Autodesk Inventor part; units mm, degrees
ref_plane "YZ Plane" through (0, 0, 0) normal (1, 0, 0) x (0, 1, 0)
ref_plane "XZ Plane" through (0, 0, 0) normal (0, 1, 0) x (-1, 0, 0)
ref_plane "XY Plane" through (0, 0, 0) normal (0, 0, 1) x (1, 0, 0)
sketch "Pole Base Profile" plane through (0, 0, 0) normal (0, 1, 0) x (-1, 0, 0)
  line L0 (3.725, 2.7) -> (-3.725, 2.7)
  line L1 (-3.725, 2.7) -> (-3.725, -2.7)
  line L2 (-3.725, -2.7) -> (3.725, -2.7)
  line L3 (3.725, -2.7) -> (3.725, 2.7)
  line L4 (3.725, 2.7) -> (-3.725, -2.7) construction
  line L5 (-3.725, 2.7) -> (3.725, -2.7) construction
  point P0 (0, 0)
  dimension "d0" = 7.45
  dimension "d1" = 5.4
extrude "Pole Base" add sketch "Pole Base Profile" along normal blind 3
sketch "Cross Base" plane through (0, 3, 0) normal (0, 1, 0) x (1, 0, 0)
  line L0 (-0.55, -2.075) -> (0.55, -2.075)
  line L1 (0.55, -2.075) -> (0.55, 2.075)
  line L2 (0.55, 2.075) -> (-0.55, 2.075)
  line L3 (-0.55, 2.075) -> (-0.55, -2.075)
  line L4 (-0.55, -2.075) -> (0.55, 2.075) construction
  line L5 (0.55, -2.075) -> (-0.55, 2.075) construction
  line L6 (-2.075, -0.55) -> (2.075, -0.55)
  line L7 (2.075, -0.55) -> (2.075, 0.55)
  line L8 (2.075, 0.55) -> (-2.075, 0.55)
  line L9 (-2.075, 0.55) -> (-2.075, -0.55)
  line L10 (-2.075, -0.55) -> (2.075, 0.55) construction
  line L11 (2.075, -0.55) -> (-2.075, 0.55) construction
  point P0 (0, 0)
  dimension "d12" = 1.1
  dimension "d13" = 4.15
  dimension "d14" = 4.15
  dimension "d15" = 1.1
extrude "Pole" add sketch "Cross Base" along normal blind 3.6
fillet "Pole Rounding" radius 0.25 8 edges at (2.075, 4.8, 0.55) (0.55, 4.8, 2.075) (-0.55, 4.8, 2.075) (-2.075, 4.8, 0.55) (-2.075, 4.8, -0.55) (-0.55, 4.8, -2.075) (0.55, 4.8, -2.075) (2.075, 4.8, -0.55)
fillet "Base Rounding" radius 0.3 4 edges at (-3.725, 3, 0) (0, 3, -2.7) (0, 3, 2.7) (3.725, 3, 0)
sketch "Top Center Point" plane through (0, 6.6, 0) normal (0, 1, 0) x (1, 0, 0)
  point P0 (0, 0)
equation "\"d0\" = s_polebl"
equation "\"d1\" = s_polebw"
equation "\"d12\" = k_cmxw"
equation "\"d13\" = k_cmxl"
equation "\"d14\" = d13"
equation "\"d15\" = d12"
equation "\"d8\" = s_poleh"
equation "\"k_width\" = 18"
equation "\"k_height\" = 16.5"
equation "\"k_taper1\" = 1.5"
equation "\"k_taper2\" = 0.5"
equation "\"k_radius\" = 6"
equation "\"k_wthick\" = 1.5"
equation "\"k_ribthick\" = 1.5"
equation "\"k_ribheight\" = 5"
equation "\"k_poleoff\" = 2.25"
equation "\"k_poledia\" = 5.3"
equation "\"k_cmxw\" = 1.1"
equation "\"k_cmxl\" = 4.15"
equation "\"s_bwidth\" = 14.4"
equation "\"s_poleh\" = 3.6"
equation "\"s_polebw\" = 5.4"
equation "\"s_polebl\" = 7.45"
equation "\"b_rshift\" = 49.5"
equation "\"b_height\" = 77"
equation "\"b_tab\" = 27"
equation "\"b_lshift\" = 40.5"
equation "\"b_space\" = 117"
equation "\"b_caps\" = 31.5"
equation "\"b_pad\" = 1"
equation "\"b_width\" = 285"
equation "\"b_ctrl\" = 22.5"
equation "\"k_staper\" = 1"
equation "\"k_ltaper\" = 1.5"
equation "\"k_sradius\" = 4"
equation "\"k_lradius\" = 6"
equation "\"k_height_t\" = 16"
equation "\"k_height_low\" = 15"
equation "\"k_taper_wide\" = 1.5"
equation "\"k_taper_thin\" = 0.0001"
equation "\"k_shortening\" = 4.5"
equation "\"k_cmxd\" = 4"
equation "\"k_taper_side\" = 0.5"
properties part number "keyswitch-pole_cherrymx"
Here's how the part is built. I have some questions about the finished solid (model axes, mm). A direction names the side the tool comes from. Round coordinates to 2 decimals unless told otherwise and drop trailing zeros. Loops run counter-clockwise (first coordinate to the right, second up) from the corner with the lowest first, then second, coordinate; pieces in that order, holes last.
1. If we section it at D-D on x = -3: Write out the boundary of the cut face in (y, z), plus the area to 3 significant figures.
Answer list:
outline: (0, -2.7) - (2.7, -2.7) arc R0.3 ccw to (3, -2.4) - (3, 2.4) arc R0.3 ccw to (2.7, 2.7) - (0, 2.7) - close
area: 16.2 mm2
2. If we section it at C-C on z = -0.05: Write out the boundary of the cut face in (x, y) (3 decimals).
Answer list:
outline: (-3.725, 0) - (3.725, 0) - (3.725, 2.7) arc R0.3 ccw to (3.425, 3) - (2.075, 3) - (2.075, 6.6) - (-2.075, 6.6) - (-2.075, 3) - (-3.425, 3) arc R0.3 ccw to (-3.725, 2.7) - close
3. Which directions (+Z, -Z, +X, -X, +Y, -Y) give clear straight access to the entire face, cutting with the end or side of a thin tool? Please do faces 1 (the face through (1, 5, -0.55)), 2 (the face through (-1, 5, 0.55)), 3 (the face through (0.55, 5, 1)), 4 (the face through (-1, 5, -0.55)), 5 (the face through (1, 3, 1)).
Answer list:
face 1: -Z, +X, +Y
face 2: +Z, -X, +Y
face 3: +Z, +X, +Y
face 4: -Z, -X, +Y
face 5: +Y
4. If we section it at B-B on y = 5: Write out the boundary of the cut face in (x, z) (3 decimals).
Answer list:
outline: (-2.075, -0.3) arc R0.25 ccw to (-1.825, -0.55) - (-0.55, -0.55) - (-0.55, -1.825) arc R0.25 ccw to (-0.3, -2.075) - (0.3, -2.075) arc R0.25 ccw to (0.55, -1.825) - (0.55, -0.55) - (1.825, -0.55) arc R0.25 ccw to (2.075, -0.3) - (2.075, 0.3) arc R0.25 ccw to (1.825, 0.55) - (0.55, 0.55) - (0.55, 1.825) arc R0.25 ccw to (0.3, 2.075) - (-0.3, 2.075) arc R0.25 ccw to (-0.55, 1.825) - (-0.55, 0.55) - (-1.825, 0.55) arc R0.25 ccw to (-2.075, 0.3) - close
5. For P1, Ø0.5, axis at y = 5, z = 0, coming from the +X side (3 decimals); P2, Ø1, axis at x = 1.5, y = 4.5, coming from the -Z side; P3, Ø3, axis at x = 0, y = 3, coming from the -Z side; P4, Ø1.5, axis at x = 0.5, y = 5.5, coming from the -Z side (3 decimals), each with a flat end and sliding along its axis, tell me the tip position at first contact or that it passes through.
Answer list:
P1: stops at x = 2.075
P2: stops at z = -0.55
P3: stops at z = -2.7
P4: stops at z = -2.075
6. If I drill on line 1 along Y through (x, z) = (-2.25, -1.15); line 2 along X through (y, z) = (4.5, 1.4), over which ranges is the centre line in solid material (lowest first)?
Answer list:
line 1: y = 0 to 3
line 2: x = -0.55 to 0.55
7. If we section it at A-A on x = 0: Write out the boundary of the cut face in (y, z) (3 decimals).
Answer list:
outline: (0, -2.7) - (2.7, -2.7) arc R0.3 ccw to (3, -2.4) - (3, -2.075) - (6.6, -2.075) - (6.6, 2.075) - (3, 2.075) - (3, 2.4) arc R0.3 ccw to (2.7, 2.7) - (0, 2.7) - close
